```python
from build123d import *

# Parameters (mm, degrees)
F0_W     = 50
F0_H     = 60
F1_DEPTH = 12.5
F2_W     = 25
F2_H     = 40
F3_DEPTH = 25.001
F4_R     = 5
F5_R     = 2


with BuildPart() as f1:
    # F0 (on Top) → F1 (new body, symmetric)
    with BuildSketch(Plane.XY):
        Rectangle(F0_W, F0_H)
    extrude(amount=F1_DEPTH, both=True)

    # F2 (on face) → F3 (cut, through all)
    with BuildSketch(Plane.XY.offset(12.5)):
        Rectangle(F2_W, F2_H)
    extrude(amount=-F3_DEPTH, mode=Mode.SUBTRACT)

    # F4
    f4_edges = [f1.edges().sort_by_distance(p)[0] for p in [
        (12.5, -20, 0),
        (-12.5, -20, 0),
        (-12.5, 20, 0),
        (12.5, 20, 0),
    ]]
    fillet(f4_edges, radius=F4_R)

    # F5
    f5_edges = [f1.edges().sort_by_distance(p)[0] for p in [
        (0, -20, 12.5),
        (-11.035534, -18.535534, 12.5),
        (11.035534, -18.535534, 12.5),
        (-12.5, 0, 12.5),
        (12.5, 0, 12.5),
        (-11.035534, 18.535534, 12.5),
        (11.035534, 18.535534, 12.5),
        (0, 20, 12.5),
        (25, 0, 12.5),
        (0, -30, 12.5),
        (0, 30, 12.5),
        (-25, 0, 12.5),
    ]]
    fillet(f5_edges, radius=F5_R)


solid = f1.part
```
Model file for the job. Use its own axes, mm. A direction names the side the tool comes from. Coordinates: 2 decimals unless noted, no trailing zeros. Write each loop counter-clockwise with the first axis right and the second up, starting at its lowest first coordinate (ties: lowest second). Pieces come first, ordered by that corner, then holes. Notation, with made-up numbers: (41, 2) - (84, 2) arc R9 cw to (84, 18) - close; hole circle Ø8 at (75.25, 76.5). An arc over 180 degrees is marked (long way). One line per item, written item: value. Start each with the question number.
1. Mould opens along X. For faces 1 (the flat face through (25, 0, -1)), 2 (the cylindrical face through (0.35, 29.43, 11.9)), 3 (the cylindrical face through (0.1, -20.57, 11.9)) say: released by +X, released by -X, zero draft, split by the parting line, or undercut.
2. Slice it at C-C (z = 1.5). Write the cut outline in (x, y).
3. Tool access for faces 4 (the flat face through (0, -30, -1)), 5 (the cylindrical face through (-13.07, -0.21, 11.9)), 6 (the cylindrical face through (11.07, 18.5, -1.16)): list every direction of +Z, -Z, +X, -X, +Y, -Y with a clear straight run to the whole face (end or side of a thin tool).
4. Slice it at A-A (y = 2.5). Write the cut outline in (x, z).
5. Probe line 1 (X direction, y = 9.5, z = 8.25); line 2 (Y direction, x = -0.5, z = -8.5); line 3 (Y direction, x = -11.5, z = 7). List the from-to ranges inside material, lowest first. Write a range as from..to.
6. Slice it at B-B (x = 1.5). Write the cut outline in (y, z).
Answers below:
1. face 1: released by +X
1. face 2: zero draft
1. face 3: undercut
2. outline: (-25, -30) - (25, -30) - (25, 30) - (-25, 30) - close; hole (-12.5, -15) arc R5 ccw to (-7.5, -20) - (7.5, -20) arc R5 ccw to (12.5, -15) - (12.5, 15) arc R5 ccw to (7.5, 20) - (-7.5, 20) arc R5 ccw to (-12.5, 15) - close
3. face 4: +Z, -Z, +X, -X, -Y
3. face 5: +Z
3. face 6: +Z, -Z
4. outline: (-25, -12.5) - (-12.5, -12.5) - (-12.5, 10.5) arc R2 ccw to (-14.5, 12.5) - (-23, 12.5) arc R2 ccw to (-25, 10.5) - close; (12.5, -12.5) - (25, -12.5) - (25, 10.5) arc R2 ccw to (23, 12.5) - (14.5, 12.5) arc R2 ccw to (12.5, 10.5) - close
5. line 1: x = -25..-12.5, 12.5..25
5. line 2: y = -30..-20, 20..30
5. line 3: y = -30..-18, 18..30
6. outline: (-30, -12.5) - (-20, -12.5) - (-20, 10.5) arc R2 ccw to (-22, 12.5) - (-28, 12.5) arc R2 ccw to (-30, 10.5) - close; (20, -12.5) - (30, -12.5) - (30, 10.5) arc R2 ccw to (28, 12.5) - (22, 12.5) arc R2 ccw to (20, 10.5) - close
